from build123d import *

# Parameters (mm, degrees)
OFFICIAL_SURFACE_TRIM_START     = -39.698691123
OFFICIAL_SURFACE_TRIM_OUTLINE_R = 25.575864924
OFFICIAL_SURFACE_TRIM_DEPTH     = 74.051423841


# Read off the part's stored shape, not the designer's step: official_surface_trim
with BuildPart() as part:
    # official_surface_trim outline → official_surface_trim (new body)
    with BuildSketch(Plane(origin=(0, 0, 0), x_dir=(1, 0, 0), z_dir=(0, 1, 0)).offset(OFFICIAL_SURFACE_TRIM_START)):
        Circle(OFFICIAL_SURFACE_TRIM_OUTLINE_R)
    extrude(amount=OFFICIAL_SURFACE_TRIM_DEPTH)


solid = part.part
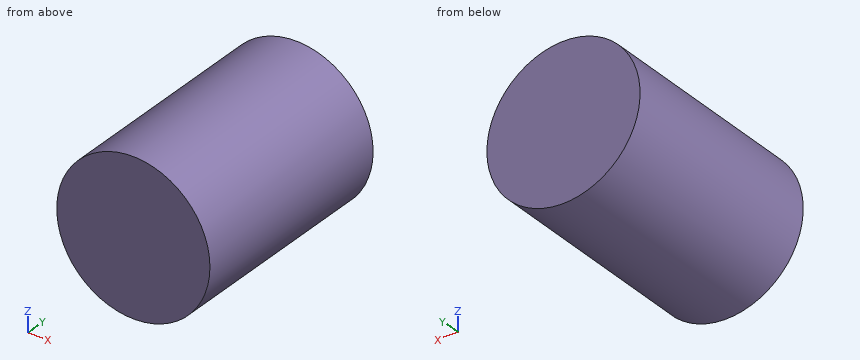
Geometry check sheet. Reference: the model listing, model coordinates, mm. Round coordinates to 2 decimals unless told otherwise and drop trailing zeros. Order: outer loops, then holes, each group sorted by start corner. A loop starts at its lowest first (then second) coordinate and runs counter-clockwise, first axis right, second up. Notation, with made-up numbers: M 35.25,68.25 L 72.25,68.25 A19 cw 72.25,87.25 Z; hole C 14.25,51.25 d11. An arc over 180 degrees is marked long. Write each question's results on one line, items separated by ' | '. Start each with the question number.
1. Cross-section at C-C on x = -20.5. Record the boundary of the cut face in (y, z), plus the area to 3 significant figures.
2. Cross-section at A-A on y = 5. Record the boundary of the cut face in (x, z), plus the area to 4 significant figures.
3. Material ranges on L1, parallel to X at y = -26.5, z = -0.5; L2, parallel to Z at x = -6, y = -31.5, recorded low to high. Write a range as from..to.
4. Go/stop test with flat-tipped pins: P1, Ø5, axis at x = 9, y = 18, coming from the +Z side; P2, Ø12, axis at x = 9.5, y = 8, coming from the -Z side; P3, Ø12, axis at y = -16, z = -12, coming from the -X side. Record where each tip stops, or that it passes through.
5. Cross-section at B-B on z = 13. Record the boundary of the cut face in (x, y), plus the area to 3 significant figures.
Resolved:
1) outline: M -39.7,-15.29 L 34.35,-15.29 L 34.35,15.29 L -39.7,15.29 Z | area: 2,260 mm2
2) outline: C 0,0 d51.15 | area: 2,055 mm2
3) L1: -25.57..25.57 | L2: -24.86..24.86
4) P1: z = 24.74 | P2: z = -25.34 | P3: x = -24.86
5) outline: M -22.03,-39.7 L 22.03,-39.7 L 22.03,34.35 L -22.03,34.35 Z | area: 3,260 mm2
